Design review of the part shown in the three views and the two pictorial views. Dimensions are in mm from the part's minimum x, y and z. A direction names the side the tool comes from. Give positions to 0.01 mm unless a question says otherwise; leave off trailing zeros. Loops run counter-clockwise (first coordinate to the right, second up) from the corner with the lowest first, then second, coordinate; pieces in that order, holes last. Notation, with made-up numbers: (32, 76.25) - (56, 76.25) arc R19 cw to (56, 98.25) - close; hole circle Ø8 at (36, -35). An arc over 180 degrees is marked (long way). Answer in a Markdown table with one row per item.
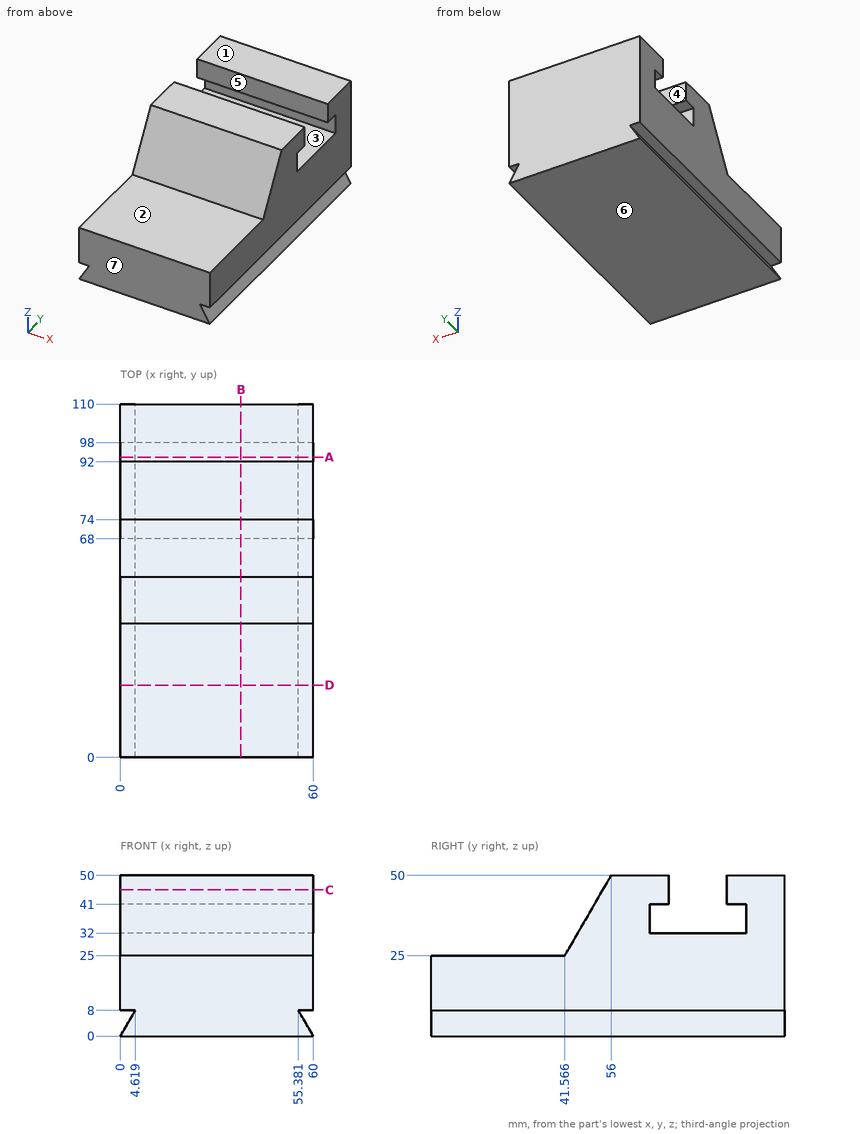
1. Clearance check with flat-ended pins moving along their axes: pin 1 (2 mm diameter, centred on x = 48.5, y = 60, fed in from -Z); pin 2 (2.5 mm diameter, centred on x = 39.5, z = 47, fed in from -Y); pin 3 (12.5 mm diameter, centred on x = 23, y = 27, fed in from +Z); pin 4 (10 mm diameter, centred on x = 21.5, z = 37, fed in from -Y). State where each tip first meets the part, or that it passes through.
Values:
| item | result |
|---|---|
| pin 1 | stops at z = 0 |
| pin 2 | stops at y = 53.55 |
| pin 3 | stops at z = 25 |
| pin 4 | stops at y = 45.61 |
2. We need section B-B, the plane x = 37.5. Give the boundary of the cut face in (y, z).
Values:
| item | result |
|---|---|
| outline | (0, 0) - (110, 0) - (110, 50) - (92, 50) - (92, 41) - (98, 41) - (98, 32) - (68, 32) - (68, 41) - (74, 41) - (74, 50) - (56, 50) - (41.57, 25) - (0, 25) - close |
3. We need section A-A, the plane y = 93.5. Give the boundary of the cut face in (x, z), and give its area (3 significant figures).
Values:
| item | result |
|---|---|
| outline | (0, 0) - (60, 0) - (55.38, 8) - (60, 8) - (60, 32) - (0, 32) - (0, 8) - (4.62, 8) - close; (0, 41) - (60, 41) - (60, 50) - (0, 50) - close |
| area | 2,420 mm^2 |
4. Wall thickness on line 1 (Z direction, x = 28, y = 71); line 2 (Z direction, x = 49.5, y = 23.5); line 3 (Z direction, x = 22, y = 79): over which ranges is each line inside the solid? List them lowest first. Write a range as [from, to].
Values:
| item | result |
|---|---|
| line 1 | z = [0, 32], [41, 50] |
| line 2 | z = [0, 25] |
| line 3 | z = [0, 32] |
5. We need section C-C, the plane z = 45.5. Give the boundary of the cut face in (x, y).
Values:
| item | result |
|---|---|
| outline | (0, 53.4) - (60, 53.4) - (60, 74) - (0, 74) - close; (0, 92) - (60, 92) - (60, 110) - (0, 110) - close |
6. Mouldability with a two-part tool opening along Y and no side actions: class the marked faces 4, 5, 6 and 7 as released by +Y, released by -Y, zero draft, split by the parting line, or undercut.
Values:
| item | result |
|---|---|
| face 4 | undercut |
| face 5 | undercut |
| face 6 | zero draft |
| face 7 | released by -Y |
7. We need section D-D, the plane y = 22.5. Give the boundary of the cut face in (x, z).
Values:
| item | result |
|---|---|
| outline | (0, 0) - (60, 0) - (55.38, 8) - (60, 8) - (60, 25) - (0, 25) - (0, 8) - (4.62, 8) - close |
8. For the marked faces 1, 2 and 3, list the 3-axis set-ups (+Z, -Z, +X, -X, +Y, -Y) from which the entire face can be reached by the end or side of a thin tool; tool diameter is ignored.
Values:
| item | result |
|---|---|
| face 1 | +Z, +X, -X, +Y, -Y |
| face 2 | +Z, +X, -X, -Y |
| face 3 | +X, -X |
